Check sheet for the modelled part. Datum: model origin and axes. Units: mm. A direction names the side the tool comes from. Give positions to 0.01 mm unless a question says otherwise; leave off trailing zeros. Order: outer loops, then holes, each group sorted by start corner. A loop starts at its lowest first (then second) coordinate and runs counter-clockwise, first axis right, second up. Notation, with made-up numbers: M 67.5,30.25 L 125.5,30.25 A35 cw 125.5,62.25 Z; hole C -28,-3.75 d10. An arc over 180 degrees is marked long. Return JSON: item names as keys, results as strings. Group by question number.
from build123d import *

# Parameters (mm, degrees)
SKETCH1_W      = 19.5
SKETCH1_H      = 20.99999991
SKETCH1_R      = 1.660700018
EXTRUDE1_DEPTH = 1.6
SKETCH2_W      = 2.54
SKETCH2_H      = 17.8
EXTRUDE2_DEPTH = 8.4


with BuildPart() as part:
    # Sketch1 → Extrude1 (new body)
    with BuildSketch(Plane(origin=(0, 0, 0), x_dir=(1, 0, 0), z_dir=(0, 1, 0))):
        with Locations((-18.583272271, -5.406568708)):
            Rectangle(SKETCH1_W, SKETCH1_H)
        with Locations(Location((-25.572572253, -13.145868645, 0), (0, 0, 270))):
            Circle(SKETCH1_R, mode=Mode.SUBTRACT)
        with Locations(Location((-25.572572253, 2.332731229, 0), (0, 0, 90))):
            Circle(SKETCH1_R, mode=Mode.SUBTRACT)
    extrude(amount=EXTRUDE1_DEPTH)

    # Sketch2 → Extrude2 (add)
    with BuildSketch(Plane.XZ):
        with Locations((-11.603272271, 5.406568708)):
            Rectangle(SKETCH2_W, SKETCH2_H)
    extrude(amount=EXTRUDE2_DEPTH)


solid = part.part
1) Sectioned sample at D-D on y = -3. Record the boundary of the cut face in (x, z).
2) Sectioned sample at C-C on z = 2. Record the boundary of the cut face in (x, y).
3) Depth check by flat-ended pin: P1, Ø1.3, axis at x = -11, y = -6, coming from the -Z side; P2, Ø4, axis at y = -4.5, z = 10.5, coming from the +X side; P3, Ø2.5, axis at y = -4, z = 4.5, coming from the -X side. Enter the tip coordinate at first touch or a pass-through.
4) Sectioned sample at B-B on x = -25.25. Record the boundary of the cut face in (y, z), then the cut area to 3 significant figures.
5) Material ranges on line 1 along Z through (x, y) = (-24.75, 0.25); line 2 along X through (y, z) = (-7.25, 9.5); line 3 along Y through (x, z) = (-21.5, 8.5), recorded low to high.
6) Tool access check on faces 1 (the face through (-12, -4, 14.307)), 2 (the face through (-10.333, -4, 5)), 3 (the face through (-12, -4, -3.493)), 4 (the face through (-19, 1, -5.093)). Record the directions out of +Z, -Z, +X, -X, +Y, -Y that give a thin tool (end or side, any length) a straight path to the whole face; none if there is none.
7) Release check for a two-part mould opening along X. For faces 5 (the face through (-24.94, 0.79, -3.87)), 6 (the face through (-12.873, -4, 5)), 7 (the face through (-19, 0, 5)) record: released by +X, released by -X, zero draft, split by the parting line, or undercut.
8) Sectioned sample at A-A on z = 13.5. Record the boundary of the cut face in (x, y), then the cut area to 3 significant figures.
Reply:
{
 "1": {"outline": "M -12.87,-3.49 L -10.33,-3.49 L -10.33,14.31 L -12.87,14.31 Z"},
 "2": {"outline": "M -28.33,0 L -12.87,0 L -12.87,-8.4 L -10.33,-8.4 L -10.33,0 L -8.83,0 L -8.83,1.6 L -28.33,1.6 Z"},
 "3": {"P1": "z = -3.49", "P2": "x = -10.33", "P3": "x = -12.87"},
 "4": {"outline": "M 0,-5.09 L 1.6,-5.09 L 1.6,-3.96 L 0,-3.96 Z; M 0,-0.7 L 1.6,-0.7 L 1.6,11.52 L 0,11.52 Z; M 0,14.77 L 1.6,14.77 L 1.6,15.91 L 0,15.91 Z", "area": "23.2 mm^2"},
 "5": {"line 1": "-5.09 to -3.78, -0.89 to 11.7, 14.59 to 15.91", "line 2": "-12.87 to -10.33", "line 3": "0 to 1.6"},
 "6": {"face 1": "+Z, +X, -X, -Y", "face 2": "+Z, -Z, +X, -Y", "face 3": "-Z, +X, -X, -Y", "face 4": "-Z, +X, -X, +Y, -Y"},
 "7": {"face 5": "undercut", "face 6": "released by -X", "face 7": "zero draft"},
 "8": {"outline": "M -28.33,0 L -27.2,0 L -27.2,1.6 L -28.33,1.6 Z; M -23.95,0 L -12.87,0 L -12.87,-8.4 L -10.33,-8.4 L -10.33,0 L -8.83,0 L -8.83,1.6 L -23.95,1.6 Z", "area": "47.3 mm^2"}
}
